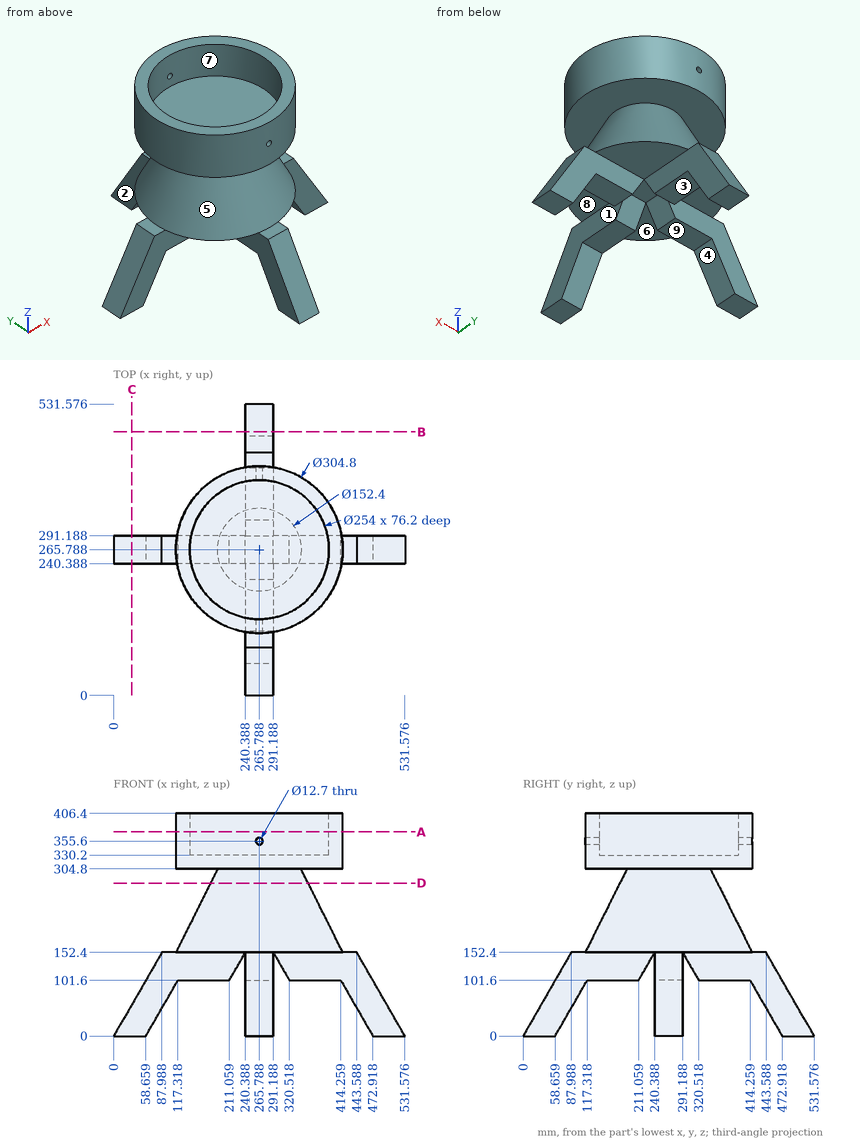
The drawing under review shows one solid part. Ordinate dimensions are in mm from its lowest x, y, z. A direction names the side the tool comes from. Coordinates: 2 decimals unless noted, no trailing zeros. Write each loop counter-clockwise with the first axis right and the second up, starting at its lowest first coordinate (ties: lowest second). Pieces come first, ordered by that corner, then holes. Notation, with made-up numbers: (47, 23) - (58, 23) arc R18 cw to (58, 56) - close; hole circle Ø8 at (66, -35.5). An arc over 180 degrees is marked (long way). Answer as CSV lines item,"result".
(1) We need section A-A (z = 372.5). Give the boundary of the cut face in (x, y), plus the area to 3 significant figures.
Data:
outline,"circle Ø304.8 at (265.79, 265.79); hole circle Ø254 at (265.79, 265.79)"
area,"22,300 mm2"
(2) We need section C-C (x = 33). Give the boundary of the cut face in (y, z), plus the area to 3 significant figures.
Data:
outline,"(240.39, 0) - (291.19, 0) - (291.19, 57.16) - (240.39, 57.16) - close"
area,"2,900 mm2"
(3) Tool access review of the marked faces 5, 6, 7, 8 and 9: name each direction out of +Z, -Z, +X, -X, +Y, -Y from which nothing blocks a thin tool from reaching the whole face with its end or side.
Data:
face 5,"none"
face 6,"-Z, -X, -Y"
face 7,"+Z"
face 8,"-Z, +X, -Y"
face 9,"-Z, +Y, -Y"
(4) We need section B-B (y = 480.5). Give the boundary of the cut face in (x, z).
Data:
outline,"(240.39, 0) - (291.19, 0) - (291.19, 88.47) - (240.39, 88.47) - close"
(5) For line 1 along Z through (x, y) = (154, 250) (1 decimal); line 2 along X through (y, z) = (275, 35.5) (1 decimal); line 3 along X through (y, z) = (284, 139.5) (1 decimal), list the stretches that pass through material, from the lowest coordinate up. Write a range as [from, to].
Data:
line 1,"z = [101.6, 231.4], [304.8, 330.2]"
line 2,"x = [20.5, 79.2], [452.4, 511.1]"
line 3,"x = [80.5, 232.9], [298.6, 451]"
(6) We need section D-D (z = 279). Give the boundary of the cut face in (x, y), plus the area to 3 significant figures.
Data:
outline,"circle Ø178.2 at (265.79, 265.79)"
area,"24,900 mm2"
(7) Clearance check with flat-ended pins moving along their axes: pin 1 Ø6 at (y, z) = (306.5, 291.5) entering from -X (1 decimal); pin 2 Ø14 at (x, y) = (257, 107) entering from +Z; pin 3 Ø5 at (y, z) = (206, 343.5) entering from -X (1 decimal); pin 4 Ø3 at (y, z) = (131, 151.5) entering from -X. State where each tip first meets the part, or that it passes through.
Data:
pin 1,"stops at x = 191.3"
pin 2,"stops at z = 406.4"
pin 3,"stops at x = 124.6"
pin 4,"stops at x = 192.44"
(8) Mouldability with a two-part tool opening along X and no side actions: class the marked faces 1, 2, 3 and 4 as pulls with the +X half, pulls with the -X half, needs draft (parallel to the pull), parting line crosses it, or undercut.
Data:
face 1,"pulls with the +X half"
face 2,"pulls with the -X half"
face 3,"needs draft"
face 4,"undercut"
